```python
from build123d import *

# Parameters (mm, degrees)
F0_W     = 7.62
F0_H     = 15.24
F1_DEPTH = 5.08
F2_R     = 1.27
F3_DEPTH = 2.54
F4_DEPTH = 15.24


# Not quite as in the source:
# - ends of sketch curves that miss each other by under 0.0002 mm in the source are joined


with BuildPart() as f1:
    # F0 (on Right) → F1 (new body)
    with BuildSketch(Plane.YZ):
        Polygon((9.5176697043, 34.8342186189), (3.1676697043, 34.8342186189), (-6.3573302957, 11.2877884223), (-0.0073302957, 11.2877884223), align=None)
        with BuildLine():
            ThreePointArc((4.4376274036, 50.074186893), (8.2142139606, 42.8663955151), (9.5176697043, 34.8342186189))
            Line((9.5176697043, 34.8342186189), (9.5176697043, 50.0742186189))
            Line((9.5176697043, 50.0742186189), (4.4376274036, 50.074186893))
        make_face()
        with Locations((13.3276697043, 42.4542186189)):
            Rectangle(F0_W, F0_H)
        Polygon((-48.9023302957, 50.0742186189), (-48.9023302957, 34.8342186189), (-41.2823302957, 34.8342186189), (-41.28180154, 34.8342186189), (-41.28180154, 50.0742186189), align=None)
        with BuildLine():
            Line((-41.28180154, 50.0742186189), (-41.28180154, 34.8342186189))
            ThreePointArc((-41.28180154, 34.8342186189), (-39.9783395258, 42.8664143264), (-36.2017354445, 50.0742186189))
            Line((-36.2017354445, 50.0742186189), (-41.28180154, 50.0742186189))
        make_face()
        Polygon((-41.28180154, 34.8342186189), (-41.2823302957, 34.8342186189), (-31.7573302957, 11.2877884223), (-25.4073302957, 11.2877884223), (-34.9323302957, 34.8342186189), align=None)
        with BuildLine():
            ThreePointArc((-13.3423302957, 60.1066603814), (-15.8823316277, 60.2339542396), (-18.4223302957, 60.1066072389))
            Line((-18.4223302957, 60.1066072389), (-18.4223302957, 57.6942186189))
            Line((-18.4223302957, 57.6942186189), (-13.3423302957, 57.6942186189))
            Line((-13.3423302957, 57.6942186189), (-13.3423302957, 60.1066603814))
        make_face()
        with BuildLine():
            Line((-18.4223302957, 62.7742186189), (-18.4223302957, 60.1066072389))
            ThreePointArc((-18.4223302957, 60.1066072389), (-15.8823316277, 60.2339542396), (-13.3423302957, 60.1066603814))
            Line((-13.3423302957, 60.1066603814), (-13.3423302957, 62.7742186189))
            Line((-13.3423302957, 62.7742186189), (-18.4223302957, 62.7742186189))
        make_face()
        with BuildLine():
            ThreePointArc((-36.2017354445, 50.0742186189), (-39.9783395258, 42.8664143264), (-41.28180154, 34.8342186189))
            Line((-41.28180154, 34.8342186189), (-34.9323302957, 34.8342186189))
            ThreePointArc((-34.9323302957, 34.8342186189), (-15.8823302957, 53.7607736673), (3.1676697043, 34.8342186189))
            Line((3.1676697043, 34.8342186189), (9.5176697043, 34.8342186189))
            ThreePointArc((9.5176697043, 34.8342186189), (8.2142139606, 42.8663955151), (4.4376274036, 50.074186893))
            ThreePointArc((4.4376274036, 50.074186893), (-3.4000386794, 56.9553751368), (-13.3423302957, 60.1066603814))
            Line((-13.3423302957, 60.1066603814), (-13.3423302957, 57.6942186189))
            Line((-13.3423302957, 57.6942186189), (-18.4223302957, 57.6942186189))
            Line((-18.4223302957, 57.6942186189), (-18.4223302957, 60.1066072389))
            ThreePointArc((-18.4223302957, 60.1066072389), (-28.3643072986, 56.9552543041), (-36.2017354445, 50.0742186189))
        make_face()
    extrude(amount=F1_DEPTH)

    # F2 (on face) → F3 (join)
    with BuildSketch(Plane.XY.offset(62.7742186189)):
        with Locations((2.54, -15.8823302957)):
            Circle(F2_R)
    extrude(amount=F3_DEPTH)

    # F0 (on Right) → F4 (join)
    with BuildSketch(Plane.YZ):
        Polygon((-48.9023302957, 50.0742186189), (-48.9023302957, 34.8342186189), (-41.2823302957, 34.8342186189), (-41.28180154, 34.8342186189), (-41.28180154, 50.0742186189), align=None)
        with BuildLine():
            Line((-41.28180154, 50.0742186189), (-41.28180154, 34.8342186189))
            ThreePointArc((-41.28180154, 34.8342186189), (-39.9783395258, 42.8664143264), (-36.2017354445, 50.0742186189))
            Line((-36.2017354445, 50.0742186189), (-41.28180154, 50.0742186189))
        make_face()
        with BuildLine():
            ThreePointArc((-36.2017354445, 50.0742186189), (-39.9783395258, 42.8664143264), (-41.28180154, 34.8342186189))
            Line((-41.28180154, 34.8342186189), (-34.9323302957, 34.8342186189))
            ThreePointArc((-34.9323302957, 34.8342186189), (-15.8823302957, 53.7607736673), (3.1676697043, 34.8342186189))
            Line((3.1676697043, 34.8342186189), (9.5176697043, 34.8342186189))
            ThreePointArc((9.5176697043, 34.8342186189), (8.2142139606, 42.8663955151), (4.4376274036, 50.074186893))
            ThreePointArc((4.4376274036, 50.074186893), (-3.4000386794, 56.9553751368), (-13.3423302957, 60.1066603814))
            Line((-13.3423302957, 60.1066603814), (-13.3423302957, 57.6942186189))
            Line((-13.3423302957, 57.6942186189), (-18.4223302957, 57.6942186189))
            Line((-18.4223302957, 57.6942186189), (-18.4223302957, 60.1066072389))
            ThreePointArc((-18.4223302957, 60.1066072389), (-28.3643072986, 56.9552543041), (-36.2017354445, 50.0742186189))
        make_face()
        with BuildLine():
            ThreePointArc((4.4376274036, 50.074186893), (8.2142139606, 42.8663955151), (9.5176697043, 34.8342186189))
            Line((9.5176697043, 34.8342186189), (9.5176697043, 50.0742186189))
            Line((9.5176697043, 50.0742186189), (4.4376274036, 50.074186893))
        make_face()
        with Locations((13.3276697043, 42.4542186189)):
            Rectangle(F0_W, F0_H)
        with BuildLine():
            ThreePointArc((-13.3423302957, 60.1066603814), (-15.8823316277, 60.2339542396), (-18.4223302957, 60.1066072389))
            Line((-18.4223302957, 60.1066072389), (-18.4223302957, 57.6942186189))
            Line((-18.4223302957, 57.6942186189), (-13.3423302957, 57.6942186189))
            Line((-13.3423302957, 57.6942186189), (-13.3423302957, 60.1066603814))
        make_face()
    extrude(amount=F4_DEPTH)


solid = f1.part
```
Geometry: final body of the model. Coordinates: model frame, mm. A direction names the side the tool comes from. Coordinates: 2 decimals unless noted, no trailing zeros. Loops run counter-clockwise (first coordinate to the right, second up) from the corner with the lowest first, then second, coordinate; pieces in that order, holes last. Notation, with made-up numbers: (-6, 23.5) -> (51, 23.5) arc R13 ccw to (51, 34.5) -> close; hole circle Ø2 at (72, 17.5). An arc over 180 degrees is marked (long way). Use a Markdown table: item, result. Add a question column.
(1) Access query for faces 1 (the cylindrical face through (1.604, -15.024, 64.026)), 2 (the flat face through (9, -42, 34.834)), 3 (the flat face through (3, -18.422, 61)), 4 (the flat face through (0, -23.4, 52.4)), 5 (the flat face through (5.08, -33, 23)). Directions: +Z, -Z, +X, -X, +Y, -Y. A direction counts if a zero-diameter tool reaches every point of the face in a straight line with its end or side. Return the directions, or none.
(2) Section query D-D, the plane y = -37. Return loops of the section in (x, z), plus the area to 3 significant figures.
(3) Section query C-C, the plane z = 51. Return loops of the section in (x, y), plus the area to 3 significant figures.
(4) Mould query, pull axis Y, two halves, no side actions, for faces 6 (the cylindrical face through (7.513, -16.3, 53.756)), 7 (the flat face through (3, -13.342, 61)), 8 (the flat face through (2.504, -1.528, 23.226)), 9 (the cylindrical face through (7.51, -15.55, 60.23)). Classes: pulls with the +Y half, pulls with the -Y half, needs draft (parallel to the pull), parting line crosses it, or undercut.
(5) Section query B-B, the plane x = 2.54. Return loops of the section in (y, z).
(6) Section query A-A, the plane z = 36. Return loops of the section in (x, y), plus the area to 3 significant figures.
(7) Line query: line 1 along X through (y, z) = (-32.5, 27); line 2 along Z through (x, y) = (10, -45); line 3 along Y through (x, z) = (10.75, 43.5). Output: solid intervals per line, ascending.
(8) Pin query (flat end, axial travel): pin 1 Ø3 at (x, y) = (13, -14.5) entering from -Z; pin 2 Ø1 at (x, y) = (6.5, -20.5) entering from +Z; pin 3 Ø0.8 at (x, z) = (1.5, 62) entering from -Y. Return the tip coordinate at first contact, or that it passes through.
Answer:
| question | item | result |
|---|---|---|
| 1 | face 1 | +Z |
| 1 | face 2 | -Z, +X, -Y |
| 1 | face 3 | +Z, +X, -X, -Y |
| 1 | face 4 | +Z, -Z, -X, +Y, -Y |
| 1 | face 5 | -Z, +X, +Y, -Y |
| 2 | outline | (0, 24.25) -> (5.08, 24.25) -> (5.08, 34.83) -> (15.24, 34.83) -> (15.24, 50.07) -> (0, 50.07) -> close |
| 2 | area | 286 mm^2 |
| 3 | outline | (0, -35.47) -> (15.24, -35.47) -> (15.24, -25.76) -> (0, -25.76) -> close; (0, -6) -> (15.24, -6) -> (15.24, 3.71) -> (0, 3.71) -> close |
| 3 | area | 296 mm^2 |
| 4 | face 6 | undercut |
| 4 | face 7 | pulls with the +Y half |
| 4 | face 8 | undercut |
| 4 | face 9 | parting line crosses it |
| 5 | outline | (-48.9, 34.83) -> (-41.28, 34.83) -> (-31.76, 11.29) -> (-25.41, 11.29) -> (-34.93, 34.83) arc R19.05 cw to (3.17, 34.83) -> (-6.36, 11.29) -> (-0.01, 11.29) -> (9.52, 34.83) -> (17.14, 34.83) -> (17.14, 50.07) -> (9.52, 50.07) -> (4.44, 50.07) arc R25.4 ccw to (-13.34, 60.11) -> (-13.34, 62.77) -> (-14.61, 62.77) -> (-14.61, 65.31) -> (-17.15, 65.31) -> (-17.15, 62.77) -> (-18.42, 62.77) -> (-18.42, 60.11) arc R25.4 ccw to (-36.2, 50.07) -> (-48.9, 50.07) -> close |
| 6 | outline | (0, -48.9) -> (15.24, -48.9) -> (15.24, -34.89) -> (0, -34.89) -> close; (0, 3.12) -> (15.24, 3.12) -> (15.24, 17.14) -> (0, 17.14) -> close |
| 6 | area | 427 mm^2 |
| 7 | line 1 | x = 0 to 5.08 |
| 7 | line 2 | z = 34.83 to 50.07 |
| 7 | line 3 | y = -48.9 to -32.78, 1.02 to 17.14 |
| 8 | pin 1 | stops at z = 53.54 |
| 8 | pin 2 | stops at z = 59.9 |
| 8 | pin 3 | stops at y = -18.42 |
